Geometry check sheet. Reference: the model listing, model coordinates, mm. A direction names the side the tool comes from. Coordinates: 2 decimals unless noted, no trailing zeros. Loops run counter-clockwise (first coordinate to the right, second up) from the corner with the lowest first, then second, coordinate; pieces in that order, holes last. Notation, with made-up numbers: (40, 58) - (97, 58) arc R15 ccw to (97, 76) - close; hole circle Ø6 at (52.5, -8). An arc over 180 degrees is marked (long way). One line per item, written item: value.
from build123d import *

# Parameters (mm, degrees)
SKETCH_1_W      = 180
SKETCH_1_H      = 120
EXTRUDE_1_DEPTH = 1
SKETCH_2_W      = 12.985294312
SKETCH_2_H      = 8.457960927
SKETCH_2_W_2    = 16.701200635
SKETCH_2_H_2    = 9.980115798
SKETCH_2_W_3    = 11.334837972
SKETCH_2_H_3    = 9.873617341
SKETCH_2_W_4    = 49.777064572
SKETCH_2_H_4    = 15.269655747
EXTRUDE_2_DEPTH = 3
SKETCH_3_R      = 5.164314182
SKETCH_3_R_2    = 7.724932849
SKETCH_3_R_3    = 10.233859985
EXTRUDE_3_DEPTH = 6


with BuildPart() as part:
    # 草图1 → 凸台-拉伸1 (new body)
    with BuildSketch(Plane(origin=(0, 0, 0), x_dir=(1, 0, 0), z_dir=(0, 1, 0))):
        Rectangle(SKETCH_1_W, SKETCH_1_H)
    extrude(amount=EXTRUDE_1_DEPTH)

    # 草图2 → 凸台-拉伸2 (add)
    with BuildSketch(Plane(origin=(0, 1, 0), x_dir=(1, 0, 0), z_dir=(0, 1, 0))):
        with Locations((-65.761091414, 32.109327308)):
            Rectangle(SKETCH_2_W, SKETCH_2_H)
        with Locations((-67.619044575, -35.458648807)):
            Rectangle(SKETCH_2_W_2, SKETCH_2_H_2)
        with Locations((-29.284234399, 8.367215504)):
            Rectangle(SKETCH_2_W_3, SKETCH_2_H_3)
        with Locations((61.715173055, 43.973135646)):
            Rectangle(SKETCH_2_W_4, SKETCH_2_H_4)
    extrude(amount=EXTRUDE_2_DEPTH)

    # 草图3 → 凸台-拉伸3 (add)
    with BuildSketch(Plane(origin=(0, 1, 0), x_dir=(1, 0, 0), z_dir=(0, 1, 0))):
        with Locations(Location((76.981635132, -8.358638316, 0), (0, 0, 90))):
            Circle(SKETCH_3_R)
        with Locations(Location((76.981635132, -40.295684365, 0), (0, 0, 90))):
            Circle(SKETCH_3_R_2)
        with Locations(Location((16.847486271, -40.295684365, 0), (0, 0, 90))):
            Circle(SKETCH_3_R_3)
    extrude(amount=EXTRUDE_3_DEPTH)


solid = part.part
(1) Cross-section at C-C on x = 51. Record the cut outline in (y, z), and give its area (3 significant figures).
Reply:
outline: (0, -60) - (1, -60) - (1, -51.61) - (4, -51.61) - (4, -36.34) - (1, -36.34) - (1, 60) - (0, 60) - close
area: 166 mm2
(2) Cross-section at D-D on x = -56.5. Record the cut outline in (y, z), and give its area (3 significant figures).
Reply:
outline: (0, -60) - (1, -60) - (1, 60) - (0, 60) - close
area: 120 mm2
(3) Cross-section at B-B on z = -7. Record the cut outline in (x, y), and give its area (3 significant figures).
Reply:
outline: (-90, 0) - (90, 0) - (90, 1) - (-23.62, 1) - (-23.62, 4) - (-34.95, 4) - (-34.95, 1) - (-90, 1) - close
area: 214 mm2
(4) Material ranges on probe 1 along Y at (x, z) = (-33.5, -30.5); probe 2 along X at (y, z) = (3.75, 41.5); probe 3 along Z at (x, y) = (-24, 2), recorded low to high. Write a range as from..to.
Reply:
probe 1: 0..1
probe 2: 6.68..27.01, 69.35..84.61
probe 3: -13.3..-3.43
(5) Go/stop test with flat-tipped pins: pin 1 Ø0.9 at (y, z) = (3, -32.5) entering from +X; pin 2 Ø1.5 at (x, y) = (-66, 3) entering from -Z; pin 3 Ø11 at (x, z) = (-66.5, 34) entering from +Y. Record where each tip stops, or that it passes through.
Reply:
pin 1: x = -59.27
pin 2: z = -36.34
pin 3: y = 4
(6) Access from +Z, -Z, +X, -X, +Y, -Y to the whole of each face (thin tool, end or side, straight path). Record for faces 1 (the face through (70.47, 3.96, 36.14)), 2 (the face through (-68, 4, 35)), 3 (the face through (61, 4, -44)).
Reply:
face 1: +Y
face 2: +Z, -Z, -X, +Y
face 3: -Z, +X, -X, +Y
(7) Release check for a two-part mould opening along X. For faces 4 (the face through (77, 7, 40)), 5 (the face through (20.767, 3.958, 30.842)), 6 (the face through (80.12, 3.96, 12.46)) record: pulls with the +X half, pulls with the -X half, needs draft (parallel to the pull), parting line crosses it, or undercut.
Reply:
face 4: needs draft
face 5: undercut
face 6: parting line crosses it
(8) Cross-section at A-A on y = 2.25. Record the cut outline in (x, z), and give its area (3 significant figures).
Reply:
outline: (-75.97, 30.47) - (-59.27, 30.47) - (-59.27, 40.45) - (-75.97, 40.45) - close; (-72.25, -36.34) - (-59.27, -36.34) - (-59.27, -27.88) - (-72.25, -27.88) - close; (-34.95, -13.3) - (-23.62, -13.3) - (-23.62, -3.43) - (-34.95, -3.43) - close; circle Ø20.47 at (16.85, 40.3); (36.83, -51.61) - (86.6, -51.61) - (86.6, -36.34) - (36.83, -36.34) - close; circle Ø15.45 at (76.98, 40.3); circle Ø10.33 at (76.98, 8.36)
area: 1,750 mm2
